from build123d import *

# Parameters (mm, degrees)
SKETCH2_W           = 53.04
SKETCH2_H           = 11
BOSS_EXTRUDE1_DEPTH = 67
SKETCH3_R           = 4.765
CUT_EXTRUDE1_DEPTH  = 87.158235822
SKETCH4_R           = 0.795
CUT_EXTRUDE2_DEPTH  = 33.5


with BuildPart() as part:
    # Sketch2 → Boss-Extrude1 (new body)
    with BuildSketch(Plane(origin=(0, 0, 0), x_dir=(1, 0, 0), z_dir=(0, 1, 0))):
        with Locations((26.52, 5.5)):
            Rectangle(SKETCH2_W, SKETCH2_H)
    extrude(amount=BOSS_EXTRUDE1_DEPTH)

    # Sketch3 → Cut-Extrude1 (cut, through all)
    with BuildSketch(Plane(origin=(0, 67, 0), x_dir=(1, 0, 0), z_dir=(0, 1, 0))):
        with Locations(Location((47.29, 5.5, 0), (0, 0, 270))):
            Circle(SKETCH3_R)
    extrude(amount=-CUT_EXTRUDE1_DEPTH, mode=Mode.SUBTRACT)

    # Sketch4 → Cut-Extrude2 (cut)
    with BuildSketch(Plane(origin=(0, 67, 0), x_dir=(1, 0, 0), z_dir=(0, 1, 0))):
        with Locations(Location((1.5, 5.5, 0), (0, 0, 270))):
            Circle(SKETCH4_R)
    extrude(amount=-CUT_EXTRUDE2_DEPTH, mode=Mode.SUBTRACT)


solid = part.part
Check sheet for the modelled part. Datum: model origin and axes. Units: mm. Coordinates: 2 decimals unless noted, no trailing zeros. Loops run counter-clockwise (first coordinate to the right, second up) from the corner with the lowest first, then second, coordinate; pieces in that order, holes last. Notation, with made-up numbers: (17, 67) -> (54, 67) arc R6 cw to (54, 73) -> close; hole circle Ø6 at (15, 16.5). An arc over 180 degrees is marked (long way). Write item = value, one per line. Start each with the question number.
1. Material ranges on line 1 (X direction, y = 53, z = -5.5) (3 decimals); line 2 (X direction, y = 18, z = -5.5) (3 decimals); line 3 (X direction, y = 11.5, z = -9.25), recorded low to high.
2. Section check B-B on x = 47.29. Record the cut outline in (y, z) (3 decimals).
3. Depth check by flat-ended pin: P1, Ø1.3, axis at x = 1.5, z = -5.5, coming from the +Y side. Enter the tip coordinate at first touch or a pass-through.
4. Section check A-A on z = -5.5. Record the cut outline in (x, y) (3 decimals), then the cut area to 3 significant figures.
5. Section check C-C on y = 18. Record the cut outline in (x, z) (3 decimals).
6. Section check D-D on y = 45. Record the cut outline in (x, z) (3 decimals).
7. Draft check along X on faces 1 (the cylindrical face through (1.016, 50.484, -6.131)), 2 (the flat face through (0, 33, -5)), 3 (the flat face through (1.5, 33.5, -5.5)), 4 (the flat face through (20, 0, -6)). Enter one of: released by +X, released by -X, zero draft, split by the parting line, or undercut.
Responses:
q1.line_1 = 0 to 0.705, 2.295 to 42.525, 52.055 to 53.04
q1.line_2 = 0 to 42.525, 52.055 to 53.04
q1.line_3 = 0 to 44.35, 50.23 to 53.04
q2.outline = (0, -11) -> (67, -11) -> (67, -10.265) -> (0, -10.265) -> close; (0, -0.735) -> (67, -0.735) -> (67, 0) -> (0, 0) -> close
q3.P1 = 33.5
q4.outline = (0, 0) -> (42.525, 0) -> (42.525, 67) -> (2.295, 67) -> (2.295, 33.5) -> (0.705, 33.5) -> (0.705, 67) -> (0, 67) -> close; (52.055, 0) -> (53.04, 0) -> (53.04, 67) -> (52.055, 67) -> close
q4.area = 2,860 mm2
q5.outline = (0, -11) -> (53.04, -11) -> (53.04, 0) -> (0, 0) -> close; hole circle Ø9.53 at (47.29, -5.5)
q6.outline = (0, -11) -> (53.04, -11) -> (53.04, 0) -> (0, 0) -> close; hole circle Ø1.59 at (1.5, -5.5); hole circle Ø9.53 at (47.29, -5.5)
q7.face_1 = undercut
q7.face_2 = released by -X
q7.face_3 = undercut
q7.face_4 = zero draft
